Could you check a few things on this model? Use its own coordinates, in mm. A direction names the side the tool comes from. Coordinates: 2 decimals unless noted, no trailing zeros. Write each loop counter-clockwise with the first axis right and the second up, starting at its lowest first coordinate (ties: lowest second). Pieces come first, ordered by that corner, then holes.
Item 1: I want a section at B-B on z = 22.5. Please give me the cut outline in (x, y), then the cut area to 3 significant figures.
Item 2: If I drill on probe 1 along X at (y, z) = (-11.5, 89.5); probe 2 along Y at (x, z) = (25.5, 52.5); probe 3 along Z at (x, y) = (-3.2, 10.75), over which ranges is the centre line in solid material (lowest first)?
Item 3: Which directions (+Z, -Z, +X, -X, +Y, -Y) give clear straight access to the entire face, cutting with the end or side of a thin tool? Please do faces 4 (the flat face through (25, 0, 64)), 5 (the flat face through (47.58, -3.42, -46.27)), 6 (the flat face through (-62, -6.75, 8)).
Item 4: Thinking about a two-plate mould opening in Y: for faces 1 (the flat face through (-18, -6.75, 69)), 2 (the flat face through (-7, -14, 90)), 3 (the flat face through (-20, 202, 62)), which applies, +Y half, -Y half, draft (parallel to the pull), parting line (faces both ways), or undercut?
Item 5: I want a section at A-A on y = 131. Please give me the cut outline in (x, z), then the cut area to 3 significant figures.
Item 6: I want a section at C-C on z = -26.5. Please give me the cut outline in (x, y).
Item 7: For P1, Ø1, axis at x = -13.5, y = 170.5, coming from the -Z side; P2, Ø5.5, axis at y = -2.5, z = 61.5, coming from the -X side; P3, Ø5, axis at x = -27, y = 13.5, coming from the -Z side, each with a flat end and sliding along its axis, tell me the tip position at first contact or that it passes through.
from build123d import *
from build123d.topology import SkipClean

# Parameters (mm, degrees)
SKETCH1_R                = 75
SKETCH1_R_2              = 57.5
BOSS_EXTRUDE1_DEPTH      = 15
BOSS_EXTRUDE2_DEPTH      = 30
BOSS_EXTRUDE2_DEPTH_BACK = 5
SKETCH2_W                = 14
SKETCH2_H                = 15
SKETCH5_W                = 2
SKETCH5_H                = 47.50869631
CUT_EXTRUDE2_DEPTH       = 64
SKETCH6_R                = 2
CUT_EXTRUDE3_DEPTH       = 64
BOSS_EXTRUDE3_DEPTH      = 6.75
BOSS_EXTRUDE4_START      = 15
BOSS_EXTRUDE4_DEPTH      = 15
SKETCH10_R               = 2
CUT_EXTRUDE5_DEPTH       = 135.989119932
SKETCH11_W               = 20
SKETCH11_H               = 6.75
CUT_EXTRUDE6_DEPTH       = 135.384011326
BOSS_EXTRUDE5_DEPTH      = 6.75
CUT_EXTRUDE8_DEPTH       = 135.166174947
BOSS_EXTRUDE6_DEPTH      = 187


with BuildPart() as part:
    # Sketch1 → Boss-Extrude1 (new body)
    with BuildSketch(Plane(origin=(0, 0, 0), x_dir=(1, 0, 0), z_dir=(0, 1, 0))):
        with Locations(Location((0, 0, 0), (0, 0, 270))):
            Circle(SKETCH1_R)
        with Locations(Location((0, 0, 0), (0, 0, 270))):
            Circle(SKETCH1_R_2, mode=Mode.SUBTRACT)
    extrude(amount=BOSS_EXTRUDE1_DEPTH)

    # Sketch2 → Boss-Extrude2 (add, two sides: drawn at the far end of the back side and taken through both)
    with BuildSketch(Plane.XY.offset(75).offset(-BOSS_EXTRUDE2_DEPTH_BACK)):
        with Locations((0, 7.5)):
            Rectangle(SKETCH2_W, SKETCH2_H)
    extrude(amount=BOSS_EXTRUDE2_DEPTH + BOSS_EXTRUDE2_DEPTH_BACK)

    # Sketch5 → Cut-Extrude2 (cut)
    with BuildSketch(Plane.XZ):
        with Locations((0, 81.245651845)):
            Rectangle(SKETCH5_W, SKETCH5_H)
    extrude(amount=-CUT_EXTRUDE2_DEPTH, mode=Mode.SUBTRACT)

    # Sketch6 → Cut-Extrude3 (cut)
    with BuildSketch(Plane(origin=(7, 0, 0), x_dir=(0, 0, -1), z_dir=(1, 0, 0))):
        with Locations(Location((-99, 4.25, 0), (0, 0, 90))):
            Circle(SKETCH6_R)
        with Locations(Location((-99, 10.75, 0), (0, 0, 90))):
            Circle(SKETCH6_R)
    extrude(amount=-CUT_EXTRUDE3_DEPTH, mode=Mode.SUBTRACT)

    # Sketch7 → Boss-Extrude3 (add)
    with BuildSketch(Plane.XZ):
        Polygon((1, 67.497826046), (1, 57.497826046), (11, 57.497826046), (11, 67.497826046), (6, 67.497826046), (6, 97.497826046), (1, 97.497826046), align=None)
        Polygon((-6, 67.49130369), (-6, 97.49130369), (-1, 97.49130369), (-1, 57.49130369), (-10.5, 57.49130369), (-10.5, 67.49130369), align=None)
    extrude(amount=BOSS_EXTRUDE3_DEPTH)

    # Sketch8 → Boss-Extrude4 (add)
    with BuildSketch(Plane.XZ.offset(6.75).offset(BOSS_EXTRUDE4_START)):
        with BuildLine():
            Line((-1, 57.50434569), (-1, 105))
            Line((-1, 105), (-7, 105))
            Line((-7, 105), (-7, 74.67261881))
            ThreePointArc((-7, 74.67261881), (0, -75), (7, 74.67261881))
            Line((7, 74.67261881), (7, 105))
            Line((7, 105), (1, 105))
            Line((1, 105), (1, 57.50434569))
            ThreePointArc((1, 57.50434569), (0, -57.513040028), (-1, 57.50434569))
        make_face()
    extrude(amount=-BOSS_EXTRUDE4_DEPTH)

    # Sketch10 → Cut-Extrude5 (cut, through all)
    with BuildSketch(Plane.ZY.offset(7)):
        with Locations((99, -10.75)):
            Circle(SKETCH10_R)
        with Locations((99, -17.75)):
            Circle(SKETCH10_R)
    extrude(amount=-CUT_EXTRUDE5_DEPTH, mode=Mode.SUBTRACT)

    # Sketch11 → Cut-Extrude6 (cut, through all)
    with BuildSketch(Plane.ZY.offset(6)):
        with Locations((87.49130369, -3.375)):
            Rectangle(SKETCH11_W, SKETCH11_H)
    extrude(amount=-CUT_EXTRUDE6_DEPTH, mode=Mode.SUBTRACT)

    # Sketch12 → Boss-Extrude5 (add)
    with SkipClean():  # the faces are left unmerged after this step: merging them gives an invalid solid
        with BuildSketch(Plane(origin=(0, -6.75, 0), x_dir=(1, 0, 0), z_dir=(0, 1, 0))):
            with BuildLine():
                Line((52.286531011, -53.769123806), (40.086340442, -41.222994918))
                ThreePointArc((40.086340442, -41.222994918), (45.124076801, -35.638009104), (49.389727695, -29.443247073))
                Line((49.389727695, -29.443247073), (64.42138395, -38.404235313))
                ThreePointArc((64.42138395, -38.404235313), (58.857491479, -46.484359701), (52.286531011, -53.769123806))
            make_face()
            with BuildLine():
                Line((-53.769123806, -52.286531011), (-41.222994918, -40.086340442))
                ThreePointArc((-41.222994918, -40.086340442), (-35.638009104, -45.124076801), (-29.443247073, -49.389727695))
                Line((-29.443247073, -49.389727695), (-38.404235313, -64.42138395))
                ThreePointArc((-38.404235313, -64.42138395), (-46.484359701, -58.857491479), (-53.769123806, -52.286531011))
            make_face()
            with BuildLine():
                Line((-52.286531011, 53.769123806), (-40.086340442, 41.222994918))
                ThreePointArc((-40.086340442, 41.222994918), (-45.124076801, 35.638009104), (-49.389727695, 29.443247073))
                Line((-49.389727695, 29.443247073), (-64.42138395, 38.404235313))
                ThreePointArc((-64.42138395, 38.404235313), (-58.857491479, 46.484359701), (-52.286531011, 53.769123806))
            make_face()
            with BuildLine():
                Line((53.769123806, 52.286531011), (41.222994918, 40.086340442))
                ThreePointArc((41.222994918, 40.086340442), (35.638009104, 45.124076801), (29.443247073, 49.389727695))
                Line((29.443247073, 49.389727695), (38.404235313, 64.42138395))
                ThreePointArc((38.404235313, 64.42138395), (46.484359701, 58.857491479), (53.769123806, 52.286531011))
            make_face()
        extrude(amount=BOSS_EXTRUDE5_DEPTH)

    # Sketch15 → Cut-Extrude8 (cut, through all)
    with SkipClean():  # the faces are left unmerged after this step: merging them gives an invalid solid
        with BuildSketch(Plane(origin=(0, 15, 0), x_dir=(1, 0, 0), z_dir=(0, 1, 0))):
            with BuildLine():
                Line((-1, -83.17261881), (-1, -79.17261881))
                ThreePointArc((-1, -79.17261881), (-3, -81.17261881), (-1, -83.17261881))
            make_face()
            with BuildLine():
                Line((1, -83.17261881), (1, -79.17261881))
                ThreePointArc((1, -79.17261881), (3, -81.17261881), (1, -83.17261881))
            make_face()
        extrude(amount=-CUT_EXTRUDE8_DEPTH, mode=Mode.SUBTRACT)

    # Sketch16 → Boss-Extrude6 (add)
    with BuildSketch(Plane(origin=(0, 15, 0), x_dir=(1, 0, 0), z_dir=(0, 1, 0))):
        with BuildLine():
            Line((-1, -74.993333037), (-1, -57.49130369))
            ThreePointArc((-1, -57.49130369), (-15.364513565, -55.409220559), (-28.75, -49.796460718))
            Line((-28.75, -49.796460718), (-37.5, -64.951905284))
            ThreePointArc((-37.5, -64.951905284), (-19.89397064, -72.313414607), (-1, -74.993333037))
        make_face()
        with BuildLine():
            Line((1, -74.993333037), (1, -57.49130369))
            ThreePointArc((1, -57.49130369), (15.364513565, -55.409220559), (28.75, -49.796460718))
            Line((28.75, -49.796460718), (37.5, -64.951905284))
            ThreePointArc((37.5, -64.951905284), (19.89397064, -72.313414607), (1, -74.993333037))
        make_face()
    extrude(amount=BOSS_EXTRUDE6_DEPTH)


solid = part.part
Response values:
1. outline: (-71.55, -21.75) - (-52.93, -21.75) - (-52.93, -6.75) - (-71.55, -6.75) - close; (-71.55, 0) - (-52.92, 0) - (-52.92, 15) - (-71.55, 15) - close; (52.92, 0) - (71.55, 0) - (71.55, 15) - (52.92, 15) - close; (52.93, -21.75) - (71.55, -21.75) - (71.55, -6.75) - (52.93, -6.75) - close
1. area: 1,120 mm2
2. probe 1: x = -7 to -1, 1 to 7
2. probe 2: y = -21.75 to -6.75, 0 to 202
2. probe 3: z = -74.93 to -57.41, 57.41 to 97, 101 to 105
3. face 4: none
3. face 5: +X
3. face 6: -X
4. face 1: undercut
4. face 2: draft
4. face 3: +Y half
5. outline: (-37.5, 64.95) - (-28.75, 49.8) arc R57.5 cw to (-1, 57.49) - (-1, 74.99) arc R75 ccw to start; (1, 57.49) arc R57.5 cw to (28.75, 49.8) - (37.5, 64.95) arc R75 ccw to (1, 74.99) - close
5. area: 1,180 mm2
6. outline: (-70.16, -21.75) - (-51.04, -21.75) - (-51.04, -6.75) - (-70.16, -6.75) - close; (-70.16, 0) - (-51.03, 0) - (-51.03, 15) - (-70.16, 15) - close; (51.03, 0) - (70.16, 0) - (70.16, 15) - (51.03, 15) - close; (51.04, -21.75) - (70.16, -21.75) - (70.16, -6.75) - (51.04, -6.75) - close
7. P1: stops at z = 55.77
7. P2: stops at x = -46.62
7. P3: stops at z = -70.89
